For this review, take the finished solid that the model builds, in its own axes (mm). Give positions to 0.01 mm unless a question says otherwise; leave off trailing zeros. Write each loop counter-clockwise with the first axis right and the second up, starting at its lowest first coordinate (ties: lowest second). Pieces come first, ordered by that corner, then holes.
Q1. Insertion check: P1, Ø5, axis at y = 295.5, z = 13.5, coming from the +X side; P2, Ø2, axis at y = 636.5, z = 30, coming from the +X side; P3, Ø12, axis at y = 1024.5, z = 23, coming from the +X side. Each pin has a flat end and moves straight along its axis. Give the tip position at first contact, or say it passes through.
Q2. For line 1 (X direction, y = 924, z = 3.5); line 2 (X direction, y = 952.5, z = 4.5), list the stretches that pass through material, from the lowest coordinate up.
Q3. We need section C-C (x = 150.5). Write out the cut boundary in (y, z).
Q4. We need section B-B (y = 598.5). Write out the cut boundary in (x, z).
Q5. We need section A-A (z = 9). Write out the cut boundary in (x, y) (3 decimals).
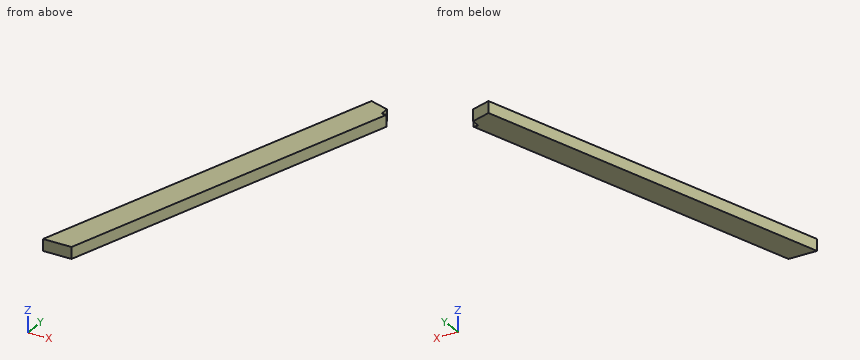
```python
from build123d import *

# Parameters (mm, degrees)
BOSS_EXTRUDE1_DEPTH = 38.1
CUT_EXTRUDE1_DEPTH  = 39.1


with BuildPart() as part:
    # Sketch2 → Boss-Extrude1 (new body)
    with BuildSketch(Plane.XY):
        Polygon((0, 0), (93.254232292, 0), (457.2, 1148.849141334), (372.450924213, 1175.696937394), align=None)
    extrude(amount=BOSS_EXTRUDE1_DEPTH)

    # Sketch3 → Cut-Extrude1 (cut, through all)
    with BuildSketch(Plane.XY.offset(38.1)):
        Polygon((434.975, 1126.624141334), (450.159306495, 1126.624141334), (457.2, 1148.849141334), (434.975, 1155.889834839), align=None)
    extrude(amount=-CUT_EXTRUDE1_DEPTH, mode=Mode.SUBTRACT)


solid = part.part
```
Computed:
1. P1: stops at x = 187.66
1. P2: stops at x = 295.21
1. P3: stops at x = 419.71
2. line 1: x = 292.72 to 385.97
2. line 2: x = 301.74 to 395
3. outline: (180.7, 0) - (475.08, 0) - (475.08, 38.1) - (180.7, 38.1) - close
4. outline: (189.6, 0) - (282.85, 0) - (282.85, 38.1) - (189.6, 38.1) - close
5. outline: (0, 0) - (93.254, 0) - (450.159, 1126.624) - (434.975, 1126.624) - (434.975, 1155.89) - (372.451, 1175.697) - close
